Read the model definition and answer for the solid it produces. Units are mm, in the model's axes. Face numbers are marked on the shaded views. A direction names the side the tool comes from. Coordinates: 2 decimals unless noted, no trailing zeros. Order: outer loops, then holes, each group sorted by start corner. A loop starts at its lowest first (then second) coordinate and runs counter-clockwise, first axis right, second up. Notation, with made-up numbers: (-34.75, -14.5) - (8.25, -14.5) arc R7 ccw to (8.25, -6.5) - close; hole circle Ø8 at (26.5, 32). An arc over 180 degrees is marked (long way). Write item = value, one per line.
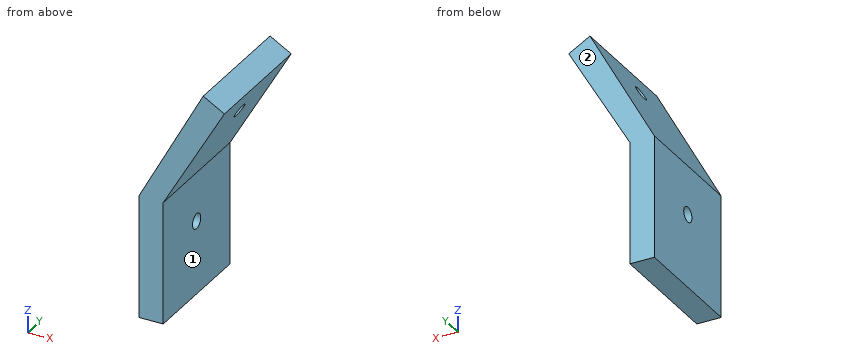
Autodesk Inventor part; units mm, degrees
ref_plane "YZ Plane" through (0, 0, 0) normal (1, 0, 0) x (0, 1, 0)
ref_plane "XZ Plane" through (0, 0, 0) normal (0, 1, 0) x (-1, 0, 0)
ref_plane "XY Plane" through (0, 0, 0) normal (0, 0, 1) x (1, 0, 0)
sketch "Sketch1" plane through (0, 0, 0) normal (0, 1, 0) x (-1, 0, 0)
  line L0 (0, 0) -> (4, 0)
  line L1 (4, 0) -> (4, -20)
  line L2 (4, -20) -> (0, -20)
  line L3 (0, -20) -> (0, 0)
  line L4 (0, 0) -> (-10, 17.3205)
  line L5 (0, 0) -> (20, 0) construction
  line L6 (-10, 17.3205) -> (-6.5359, 19.3205)
  line L7 (-6.5359, 19.3205) -> (4, 0)
  dimension "d0" = 4
  dimension "d1" = 20
  dimension "d2" = 20
  dimension "d3" = 120
  dimension "d4" = 4
extrude "Extrusion1" add sketch "Sketch1" along normal blind 20
sketch "Sketch2" plane through (0, 0, 0) normal (1, 0, 0) x (0, 0, -1)
  line L0 (0, 0) -> (0, 20)
  line L1 (0, 0) -> (20, 0)
  point P0 (8, 10)
  point P1 (0, 10)
  dimension "d7" = 8
  dimension "d8" = 10
hole "Hole1" at (0, 10, -8) direction (-1, 0, 0) diameter 2.45 end through all
sketch "Sketch3" plane through (0, 0, 0) normal (0.8660254, 0, -0.5) x (-0.5, 0, -0.8660254)
  line L0 (0, 0) -> (0, 20)
  line L1 (-20, 20) -> (0, 20)
  point P0 (-14, 10)
  point P1 (0, 10)
  dimension "d16" = 14
  dimension "d17" = 10
hole "Hole2" at (7, 10, 12.1244) direction (-0.8660254, 0, 0.5) diameter 2.45 end through all
equation "\"d0\" = d4"
properties part number "150degreebracket" material "Iron, Malleable"
1) The part is cut by section C-C (x = -2). Determine the outline of the cut face in (y, z) (3 decimals).
Returned:
outline = (0, -20) - (20, -20) - (20, 3.668) - (0, 3.668) - close; hole circle Ø2.45 at (10, -8)
2) The part is cut by section B-B (y = 10). Determine the outline of the cut face in (x, z) (1 decimal).
Returned:
outline = (-4, -20) - (0, -20) - (0, -9.2) - (-4, -9.2) - close; (-4, -6.8) - (0, -6.8) - (0, 0) - (6.4, 11.1) - (3.1, 13) - (-4, 0) - close; (4.2, 15.1) - (7.6, 13.2) - (10, 17.3) - (6.5, 19.3) - close
3) The part is cut by section D-D (y = 16). Determine the outline of the cut face in (x, z).
Returned:
outline = (-4, -20) - (0, -20) - (0, 0) - (10, 17.32) - (6.54, 19.32) - (-4, 0) - close
4) Straight lines are drawn through the part: line 1 along X through (y, z) = (12, 0); line 2 along Y through (x, z) = (-2.55, -8) (3 decimals); line 3 along Z through (x, y) = (-1.95, 10) (3 decimals). For each, find the intervals that lie inside material, in ascending order. Write a range as from..to.
Returned:
line_1 = -4..0
line_2 = 0..8.775, 11.225..20
line_3 = -20..-9.225, -6.775..3.759
5) For the marked faces 1 and 2, determine the directions among +Z, -Z, +X, -X, +Y, -Y from which every point of the face is accessible in a straight line to the end or side of a thin tool.
Returned:
face_1 = -Z, +X, +Y, -Y
face_2 = +Z, -Z, +X, -X, +Y
6) The part is cut by section A-A (z = -8). Determine the outline of the cut face in (x, y) (3 decimals), and give its area (3 significant figures).
Returned:
outline = (-4, 0) - (0, 0) - (0, 8.775) - (-4, 8.775) - close; (-4, 11.225) - (0, 11.225) - (0, 20) - (-4, 20) - close
area = 70.2 mm^2
7) Flat-ended cylindrical pins translate along their axes: pin 1 Ø2 at (x, y) = (8, 12) entering from +Z; pin 2 Ø3 at (x, y) = (6.5, 17) entering from -Z; pin 3 Ø12 at (y, z) = (3.5, -6.5) entering from +X. Find the tip coordinate at first contact, or state that the pin passes through.
Returned:
pin_1 = 19.05
pin_2 = 8.66
pin_3 = 0
